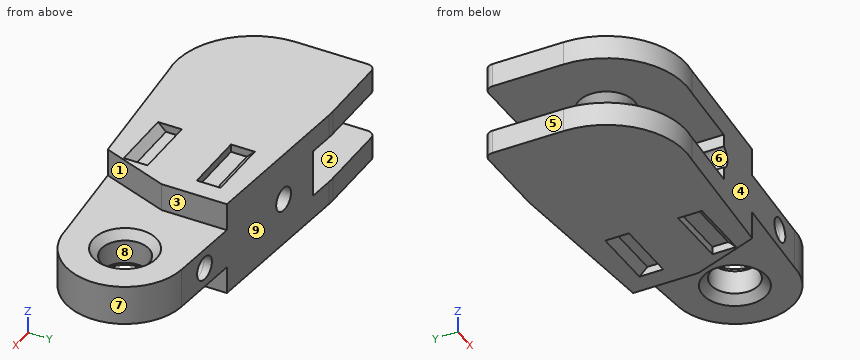
```python
from build123d import *

# Parameters (mm, degrees)
BOSS_EXTRUDE1_DEPTH  = 6
SKETCH1_3_R          = 2.5
BOSS_EXTRUDE2_DEPTH  = 6
SKETCH1_5_R          = 7.5
SKETCH1_5_R_2        = 3
BOSS_EXTRUDE3_DEPTH  = 4.5
SKETCH1_6_R          = 2.5
CUT_EXTRUDE2_DEPTH   = 3
CUT_EXTRUDE3_DEPTH   = 3
CUT_EXTRUDE4_START   = -10
CUT_EXTRUDE4_DEPTH   = 7.5
CUT_SWEEP5_PROFILE_R = 1.5
SKETCH1_7_R          = 2.5
BOSS_EXTRUDE4_DEPTH  = 6
CHAMFER1_SIZE        = 1
CUT_EXTRUDE5_DEPTH   = 4
MIRROR4_COPY_1_DEPTH = 4


with BuildPart() as part:
    # Sketch1 → Boss-Extrude1 (new, symmetric)
    with BuildSketch(Plane.XY):
        with BuildLine():
            Line((15.625, 7.473912964), (-14.166666667, 9.965217286))
            ThreePointArc((-14.166666667, 9.965217286), (-5.008579418, 0.414143408), (-13.344827586, -9.862068966))
            Line((-13.344827586, -9.862068966), (15, -7.5))
            ThreePointArc((15, -7.5), (7.506524597, 0.312772095), (15.625, 7.473912964))
        make_face()
    extrude(amount=BOSS_EXTRUDE1_DEPTH, both=True)

    # Sketch1_3 → Boss-Extrude2 (add, symmetric)
    with BuildSketch(Plane.XY):
        with BuildLine():
            Line((-15, 10), (-24, 10))
            ThreePointArc((-24, 10), (-24.707106781, 9.707106781), (-25, 9))
            Line((-25, 9), (-25, 0))
            ThreePointArc((-25, 0), (-7.928932188, -7.071067812), (-15, 10))
        make_face()
        with Locations((-15, 0)):
            Circle(SKETCH1_3_R, mode=Mode.SUBTRACT)
    extrude(amount=BOSS_EXTRUDE2_DEPTH, both=True)

    # Sketch1_5 → Boss-Extrude3 (add, symmetric)
    with BuildSketch(Plane.XY):
        with Locations((15, 0)):
            Circle(SKETCH1_5_R)
        with Locations((15, 0)):
            Circle(SKETCH1_5_R_2, mode=Mode.SUBTRACT)
    extrude(amount=BOSS_EXTRUDE3_DEPTH, both=True)

    # Sketch1_6 → Cut-Extrude2 (cut, symmetric)
    with BuildSketch(Plane.XY):
        with BuildLine():
            Line((-15, 10), (-24, 10))
            ThreePointArc((-24, 10), (-24.707106781, 9.707106781), (-25, 9))
            Line((-25, 9), (-25, 0))
            ThreePointArc((-25, 0), (-7.928932188, -7.071067812), (-15, 10))
        make_face()
        with Locations((-15, 0)):
            Circle(SKETCH1_6_R, mode=Mode.SUBTRACT)
    extrude(amount=CUT_EXTRUDE2_DEPTH, both=True, mode=Mode.SUBTRACT)

    # Sketch2 → Cut-Extrude3 (cut, symmetric)
    with BuildSketch(Plane.XY):
        with BuildLine():
            Line((-4.5, 0), (-4.5, -10.5))
            Line((-4.5, -10.5), (-15, -10.5))
            ThreePointArc((-15, -10.5), (-22.424621202, 7.424621202), (-4.5, 0))
        make_face()
    extrude(amount=CUT_EXTRUDE3_DEPTH, both=True, mode=Mode.SUBTRACT)

    # Sketch2_3 → Cut-Extrude4 (cut)
    with BuildSketch(Plane.XY.offset(CUT_EXTRUDE4_START)):
        with BuildLine():
            Line((6.475875471, 0), (3, -9.448823218))
            Line((3, -9.448823218), (15, -9.448823218))
            Line((15, -9.448823218), (15, -8))
            ThreePointArc((15, -8), (23, 0), (15, 8))
            Line((15, 8), (6.475875471, 8.877657642))
            Line((6.475875471, 8.877657642), (6.475875471, 0))
        make_face()
    cut_extrude4 = extrude(amount=CUT_EXTRUDE4_DEPTH, mode=Mode.SUBTRACT)

    # Mirror1: Cut-Extrude4 across plane
    add(cut_extrude4.mirror(Plane.XY), mode=Mode.SUBTRACT)

    # Cut-Sweep5: sweep along a path in Sketch3
    with BuildLine(Plane.XY) as cut_sweep5_path:
        Line((-5, 11.376707414), (-5, 9.19866211))
        Line((-5, 9.19866211), (-5, 7))
        ThreePointArc((-5, 7), (-4.121320344, 4.878679656), (-2, 4))
        Line((-2, 4), (8, 4))
        ThreePointArc((8, 4), (10.121320344, 4.878679656), (11, 7))
        Line((11, 7), (11, 7.860674894))
        Line((11, 7.860674894), (11, 10.978155515))
    # Cut-Sweep5 profile (on start of the path) → Cut-Sweep5 (sweep, cut)
    with BuildSketch(Plane(origin=(-5, 11.376707414, 0), x_dir=(0, 0, -1), z_dir=(0, -1, 0))):
        Circle(CUT_SWEEP5_PROFILE_R)
    cut_sweep5 = sweep(path=cut_sweep5_path.line, mode=Mode.SUBTRACT)

    # Mirror2: Cut-Sweep5 across plane
    add(cut_sweep5.mirror(Plane.ZX), mode=Mode.SUBTRACT)

    # Sketch1_7 → Boss-Extrude4 (add, symmetric)
    with BuildSketch(Plane.XY):
        with Locations((-15, 0)):
            Circle(SKETCH1_7_R)
    extrude(amount=BOSS_EXTRUDE4_DEPTH, both=True)

    # Chamfer1
    chamfer1_edges = [part.edges().sort_by_distance(p)[0] for p in [
        (12, 0, -2.5),
        (12, 0, 2.5),
        (-17.5, 0, 3),
        (-17.5, 0, -3),
    ]]
    chamfer(chamfer1_edges, length=CHAMFER1_SIZE)

    # Sketch139 → Cut-Extrude5 (cut, symmetric)
    with BuildSketch(Plane(origin=(0, 0, 0), x_dir=(0, 0, -1), z_dir=(1, 0, 0))):
        Polygon((6, 9.102109239), (6, 6.102109239), (5, 5.102109239), (5, 3.102109239), (7.604988318, 3.102109239), (7.604988318, 9.102109239), align=None)
    cut_extrude5 = extrude(amount=CUT_EXTRUDE5_DEPTH, both=True, mode=Mode.SUBTRACT)

    # Mirror3: Cut-Extrude5 across plane
    add(cut_extrude5.mirror(Plane.ZX), mode=Mode.SUBTRACT)

    # Mirror4: Cut-Extrude5 across plane
    add(cut_extrude5.mirror(Plane.XY), mode=Mode.SUBTRACT)

    # Mirror4 copy 1 sketch → Mirror4 copy 1 (cut, symmetric)
    with BuildSketch(Plane(origin=(0, 0, 0), x_dir=(0, 0, 1), z_dir=(1, 0, 0))):
        Polygon((6, 9.102109239), (6, 6.102109239), (5, 5.102109239), (5, 3.102109239), (7.604988318, 3.102109239), (7.604988318, 9.102109239), align=None)
    extrude(amount=MIRROR4_COPY_1_DEPTH, both=True, mode=Mode.SUBTRACT)


solid = part.part
```
Source: CAD feature listing. Evaluate the final solid. Frame: model axes, mm. Face numbers are marked on the shaded views. A direction names the side the tool comes from. Give positions to 0.01 mm unless a question says otherwise; leave off trailing zeros. Loops run counter-clockwise (first coordinate to the right, second up) from the corner with the lowest first, then second, coordinate; pieces in that order, holes last. Notation, with made-up numbers: (3.25, -6) -> (34.25, -6) arc R24 cw to (34.25, 11) -> close; hole circle Ø4 at (88.5, -30). An arc over 180 degrees is marked (long way). Put each result on its own line as item: value. Start each with the question number.
1) Cut plane A-A (z = 0). State how many separate pieces and enclosed holes the cut face has, then the cut area to 3 significant figures.
2) Contact query for flat-ended pins moving along their axis: P1, Ø1, axis at x = -1.5, y = 4.5, coming from the -Z side; P2, Ø4, axis at y = 3.5, z = -5, coming from the +X side; P3, Ø1.1, axis at x = 0, z = 5.5, coming from the +Y side. Output: stop coordinate, or through.
3) Cut plane B-B (x = 2). Return loops of the section in (y, z).
4) Material intervals for probe 1 along Z at (x, y) = (-5, 8.8); probe 2 along Y at (x, z) = (2.5, 0); probe 3 along Y at (x, z) = (5.75, 0), sorted ascending.
5) Cut plane D-D (x = -8). Return loops of the section in (y, z).
6) Reachability of the marked faces 1, 2, 3, 4 and 5 from +Z, -Z, +X, -X, +Y, -Y: full face, straight path, thin tool, end or side. Return the list, or none.
7) Draft query along Y for the marked faces 6, 7, 8 and 9. Return one class per face: released by +Y, released by -Y, zero draft, split by the parting line, or undercut.
Results are:
1. separate pieces: 5
1. enclosed holes: 1
1. area: 295 mm2
2. P1: stops at z = -5
2. P2: stops at x = 6.48
2. P3: stops at y = 8.83
3. outline: (-8.58, -6) -> (-6.1, -6) -> (-5.1, -5) -> (-3.1, -5) -> (-3.1, -6) -> (3.1, -6) -> (3.1, -5) -> (5.1, -5) -> (6.1, -6) -> (8.61, -6) -> (8.61, 6) -> (6.1, 6) -> (5.1, 5) -> (3.1, 5) -> (3.1, 6) -> (-3.1, 6) -> (-3.1, 5) -> (-5.1, 5) -> (-6.1, 6) -> (-8.58, 6) -> close; hole circle Ø3 at (-4, 0); hole circle Ø3 at (4, 0)
4. probe 1: z = -6 to -1.5, 1.5 to 6
4. probe 2: y = -8.54 to -5.5, -2.5 to 2.5, 5.5 to 8.57
4. probe 3: y = -8.27 to -5.5, -2.5 to 2.5, 5.5 to 8.3
5. outline: (-9.42, -6) -> (9.45, -6) -> (9.45, 6) -> (-9.42, 6) -> (-9.42, 3) -> (7.83, 3) -> (7.83, -3) -> (-9.42, -3) -> close
6. face 1: +Z, +X, -Y
6. face 2: none
6. face 3: +Z, +X, +Y, -Y
6. face 4: +Z, -Z, +X, -Y
6. face 5: +Z, -Z, -X, +Y, -Y
7. face 6: zero draft
7. face 7: split by the parting line
7. face 8: undercut
7. face 9: released by +Y
